from build123d import *

# Parameters (mm, degrees)
BOSS_EXTRUDE1_DEPTH = 6
SKETCH2_W           = 5
SKETCH2_H           = 5
CUT_EXTRUDE1_DEPTH  = 40.357337308
CUT_EXTRUDE2_DEPTH  = 40.357337308
SKETCH6_W           = 6
SKETCH6_H           = 6
CUT_EXTRUDE5_DEPTH  = 36.510561809
FILLET1_R           = 10
FILLET2_R           = 3
SKETCH5_R           = 1
CUT_EXTRUDE3_DEPTH  = 36.510561809


with BuildPart() as part:
    # Sketch1 → Boss-Extrude1 (new body)
    with BuildSketch(Plane(origin=(0, 0, 0), x_dir=(1, 0, 0), z_dir=(0, 1, 0))):
        Polygon((21, 0), (21, 9), (27, 9), (27, 28), (0, 28), (0, 0), align=None)
    extrude(amount=BOSS_EXTRUDE1_DEPTH)

    # Sketch2 → Cut-Extrude1 (cut, through all)
    with BuildSketch(Plane(origin=(0, 6, 0), x_dir=(1, 0, 0), z_dir=(0, 1, 0))):
        with Locations((5.615223689, 22.884776311)):
            Rectangle(SKETCH2_W, SKETCH2_H)
        with Locations((14.807611845, 13.692388155)):
            Rectangle(SKETCH2_W, SKETCH2_H)
    extrude(amount=-CUT_EXTRUDE1_DEPTH, mode=Mode.SUBTRACT)

    # Sketch3 → Cut-Extrude2 (cut, through all)
    with BuildSketch(Plane(origin=(0, 6, 0), x_dir=(1, 0, 0), z_dir=(0, 1, 0))):
        Polygon((21, 18), (11, 28), (33.43673633, 34.250964333), (36.08047681, 3.383507916), (21, 9), align=None)
    extrude(amount=-CUT_EXTRUDE2_DEPTH, mode=Mode.SUBTRACT)

    # Sketch6 → Cut-Extrude5 (cut, through all)
    with BuildSketch(Plane(origin=(0, 6, 0), x_dir=(1, 0, 0), z_dir=(0, 1, 0))):
        with Locations((6.115223689, 22.384776311)):
            Rectangle(SKETCH6_W, SKETCH6_H)
        with Locations((15.307611845, 13.192388155)):
            Rectangle(SKETCH6_W, SKETCH6_H)
    extrude(amount=-CUT_EXTRUDE5_DEPTH, mode=Mode.SUBTRACT)

    # Fillet1
    fillet1_edges = [part.edges().sort_by_distance(p)[0] for p in [
        (21, 3, -18),
    ]]
    fillet(fillet1_edges, radius=FILLET1_R)

    # Fillet2
    fillet2_edges = [part.edges().sort_by_distance(p)[0] for p in [
        (0, 3, -28),
        (11, 3, -28),
    ]]
    fillet(fillet2_edges, radius=FILLET2_R)

    # Sketch5 → Cut-Extrude3 (cut, through all)
    with BuildSketch(Plane(origin=(0, 6, 0), x_dir=(1, 0, 0), z_dir=(0, 1, 0))):
        with Locations(Location((5, 12, 0), (0, 0, 270))):
            Circle(SKETCH5_R)
        with Locations(Location((5, 9, 0), (0, 0, 270))):
            Circle(SKETCH5_R)
    extrude(amount=-CUT_EXTRUDE3_DEPTH, mode=Mode.SUBTRACT)


solid = part.part
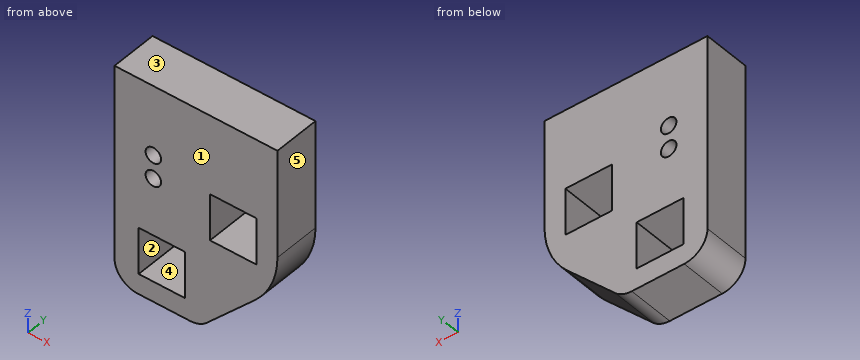
Could you check a few things on this model? Use its own coordinates, in mm. Face numbers are marked on the shaded views. A direction names the side the tool comes from. Coordinates: 2 decimals unless noted, no trailing zeros. Order: outer loops, then holes, each group sorted by start corner. A loop starts at its lowest first (then second) coordinate and runs counter-clockwise, first axis right, second up. Notation, with made-up numbers: (52.5, 89) - (99.5, 89) arc R18 cw to (99.5, 93) - close; hole circle Ø2 at (-23.75, -3.75). An arc over 180 degrees is marked (long way). Answer in a Markdown table with one row per item. Add a question column.
(1) If we section it at A-A, the plane z = -12: Please give me the cut outline in (x, y).
(2) If we section it at C-C, the plane x = 7.25: Please give me the cut outline in (y, z), then the cut area to 3 significant figures.
(3) If we mould it in two halves opening along X, with no side actions, what happens to the marked faces 3, 4 and 5? For each: released by +X, released by -X, zero draft, split by the parting line, or undercut.
(4) On a 3-axis mill with a long thin cutter (end or side, diameter ignored), from which of +Z, -Z, +X, -X, +Y, -Y can I reach the whole of each face in a straight line? I mean the marked faces 1 and 2. Say none if no direction works.
(5) Will these pins go through, and if not, where does the flat tip stop? pin 1 (2 mm diameter, centred on x = 17.5, z = -23.5, fed in from -Y); pin 2 (3 mm diameter, centred on x = 15, y = 3, fed in from -Z); pin 3 (3 mm diameter, centred on y = 3, z = -22.5, fed in from +X).
(6) If we section it at D-D, the plane z = -9: Please give me the cut outline in (x, y).
(7) I need wall thicknesses on L1, parallel to X at y = 3.6, z = -12; L2, parallel to Z at x = 3.5, y = 3; L3, parallel to X at y = 3.15, z = -9. Which ranges of each line are inside material? Lowest first, please.
(8) If we section it at B-B, the plane y = 1.5: Please give me the cut outline in (x, z).
Results are:
| question | item | result |
|---|---|---|
| 1 | outline | (0, 0) - (4, 0) - (4, 6) - (0, 6) - close; (6, 0) - (12.31, 0) - (12.31, 6) - (6, 6) - close; (18.31, 0) - (21, 0) - (21, 6) - (18.31, 6) - close |
| 2 | outline | (0, -28) - (6, -28) - (6, -25.38) - (0, -25.38) - close; (0, -19.38) - (6, -19.38) - (6, 0) - (0, 0) - close |
| 2 | area | 132 mm2 |
| 3 | face 3 | zero draft |
| 3 | face 4 | undercut |
| 3 | face 5 | released by +X |
| 4 | face 1 | +Z, -Z, +X, -X, -Y |
| 4 | face 2 | +Y, -Y |
| 5 | pin 1 | passes through |
| 5 | pin 2 | stops at z = -25.5 |
| 5 | pin 3 | stops at x = 18 |
| 6 | outline | (0, 0) - (4, 0) - (4, 6) - (0, 6) - close; (6, 0) - (21, 0) - (21, 6) - (6, 6) - close |
| 7 | L1 | x = 0 to 4, 6 to 12.31, 18.31 to 21 |
| 7 | L2 | z = -28 to -25.38, -19.38 to 0 |
| 7 | L3 | x = 0 to 4, 6 to 21 |
| 8 | outline | (0, -25) arc R3 ccw to (3, -28) - (9.76, -28) arc R3 ccw to (11.88, -27.12) - (18.07, -20.93) arc R10 ccw to (21, -13.86) - (21, 0) - (0, 0) - close; hole (3.12, -25.38) - (9.12, -25.38) - (9.12, -19.38) - (3.12, -19.38) - close; hole circle Ø2 at (5, -12); hole circle Ø2 at (5, -9); hole (12.31, -16.19) - (18.31, -16.19) - (18.31, -10.19) - (12.31, -10.19) - close |
